```python
from build123d import *

# Parameters (mm, degrees)
SKETCH1_R             = 101
SKETCH1_R_2           = 3.175
SKETCH1_R_3           = 86.77
BOSS_EXTRUDE1_DEPTH   = 6
SKETCH1_R_4           = 84.23
SKETCH1_R_5           = 70
BOSS_EXTRUDE1_2_DEPTH = 6
SKETCH1_3_R           = 86.77
SKETCH1_3_R_2         = 84.23
BOSS_EXTRUDE2_DEPTH   = 1.5875
BOSS_EXTRUDE3_START   = 6
SKETCH1_4_R           = 84.23
SKETCH1_4_R_2         = 3.175
SKETCH1_4_R_3         = 70
BOSS_EXTRUDE3_DEPTH   = 2
BOSS_EXTRUDE4_START   = -8
SKETCH1_5_R           = 101
SKETCH1_5_R_2         = 3.175
SKETCH1_5_R_3         = 86.77
BOSS_EXTRUDE4_DEPTH   = 2


with BuildPart() as part:
    # Sketch1 → Boss-Extrude1 (new, symmetric)
    with BuildSketch(Plane(origin=(0, 0, 0), x_dir=(1, 0, 0), z_dir=(0, 1, 0))):
        with Locations(Location((0, 0, 0), (0, 0, 270))):
            Circle(SKETCH1_R)
        with Locations(Location((-66.888765966, -66.888765966, 0), (0, 0, 270))):
            Circle(SKETCH1_R_2, mode=Mode.SUBTRACT)
        with Locations(Location((66.888765966, 66.888765966, 0), (0, 0, 270))):
            Circle(SKETCH1_R_2, mode=Mode.SUBTRACT)
        with Locations(Location((0, 0, 0), (0, 0, 270))):
            Circle(SKETCH1_R_3, mode=Mode.SUBTRACT)
        with Locations(Location((66.888765966, -66.888765966, 0), (0, 0, 270))):
            Circle(SKETCH1_R_2, mode=Mode.SUBTRACT)
        with Locations(Location((-66.888765966, 66.888765966, 0), (0, 0, 270))):
            Circle(SKETCH1_R_2, mode=Mode.SUBTRACT)
    extrude(amount=BOSS_EXTRUDE1_DEPTH, both=True)



with BuildPart() as body_2:
    # Sketch1 → Boss-Extrude1 2 (new, symmetric)
    with BuildSketch(Plane(origin=(0, 0, 0), x_dir=(1, 0, 0), z_dir=(0, 1, 0))):
        with Locations(Location((0, 0, 0), (0, 0, 270))):
            Circle(SKETCH1_R_4)
        with Locations(Location((-54.800775542, 54.800775542, 0), (0, 0, 270))):
            Circle(SKETCH1_R_2, mode=Mode.SUBTRACT)
        with Locations(Location((-54.800775542, -54.800775542, 0), (0, 0, 270))):
            Circle(SKETCH1_R_2, mode=Mode.SUBTRACT)
        with Locations(Location((54.800775542, -54.800775542, 0), (0, 0, 270))):
            Circle(SKETCH1_R_2, mode=Mode.SUBTRACT)
        with Locations(Location((54.800775542, 54.800775542, 0), (0, 0, 270))):
            Circle(SKETCH1_R_2, mode=Mode.SUBTRACT)
        with Locations(Location((0, 0, 0), (0, 0, 270))):
            Circle(SKETCH1_R_5, mode=Mode.SUBTRACT)
    extrude(amount=BOSS_EXTRUDE1_2_DEPTH, both=True)


with BuildPart() as part_1:
    add(part.part)

    add(body_2.part)  # Boss-Extrude2 merges body 2
    # Sketch1<3> → Boss-Extrude2 (add, symmetric)
    with BuildSketch(Plane(origin=(0, 0, 0), x_dir=(1, 0, 0), z_dir=(0, 1, 0))):
        with Locations(Location((0, 0, 0), (0, 0, 270))):
            Circle(SKETCH1_3_R)
        with Locations(Location((0, 0, 0), (0, 0, 270))):
            Circle(SKETCH1_3_R_2, mode=Mode.SUBTRACT)
    extrude(amount=BOSS_EXTRUDE2_DEPTH, both=True)

    # Sketch1<4> → Boss-Extrude3 (add)
    with BuildSketch(Plane(origin=(0, 0, 0), x_dir=(1, 0, 0), z_dir=(0, 1, 0)).offset(BOSS_EXTRUDE3_START)):
        with Locations(Location((0, 0, 0), (0, 0, 270))):
            Circle(SKETCH1_4_R)
        with Locations(Location((-54.800775542, 54.800775542, 0), (0, 0, 270))):
            Circle(SKETCH1_4_R_2, mode=Mode.SUBTRACT)
        with Locations(Location((-54.800775542, -54.800775542, 0), (0, 0, 270))):
            Circle(SKETCH1_4_R_2, mode=Mode.SUBTRACT)
        with Locations(Location((54.800775542, -54.800775542, 0), (0, 0, 270))):
            Circle(SKETCH1_4_R_2, mode=Mode.SUBTRACT)
        with Locations(Location((54.800775542, 54.800775542, 0), (0, 0, 270))):
            Circle(SKETCH1_4_R_2, mode=Mode.SUBTRACT)
        with Locations(Location((0, 0, 0), (0, 0, 270))):
            Circle(SKETCH1_4_R_3, mode=Mode.SUBTRACT)
    extrude(amount=BOSS_EXTRUDE3_DEPTH)

    # Sketch1<5> → Boss-Extrude4 (add)
    with BuildSketch(Plane(origin=(0, 0, 0), x_dir=(1, 0, 0), z_dir=(0, 1, 0)).offset(BOSS_EXTRUDE4_START)):
        with Locations(Location((0, 0, 0), (0, 0, 270))):
            Circle(SKETCH1_5_R)
        with Locations(Location((-66.888765966, -66.888765966, 0), (0, 0, 270))):
            Circle(SKETCH1_5_R_2, mode=Mode.SUBTRACT)
        with Locations(Location((66.888765966, 66.888765966, 0), (0, 0, 270))):
            Circle(SKETCH1_5_R_2, mode=Mode.SUBTRACT)
        with Locations(Location((0, 0, 0), (0, 0, 270))):
            Circle(SKETCH1_5_R_3, mode=Mode.SUBTRACT)
        with Locations(Location((66.888765966, -66.888765966, 0), (0, 0, 270))):
            Circle(SKETCH1_5_R_2, mode=Mode.SUBTRACT)
        with Locations(Location((-66.888765966, 66.888765966, 0), (0, 0, 270))):
            Circle(SKETCH1_5_R_2, mode=Mode.SUBTRACT)
    extrude(amount=BOSS_EXTRUDE4_DEPTH)


solid = part_1.part
```
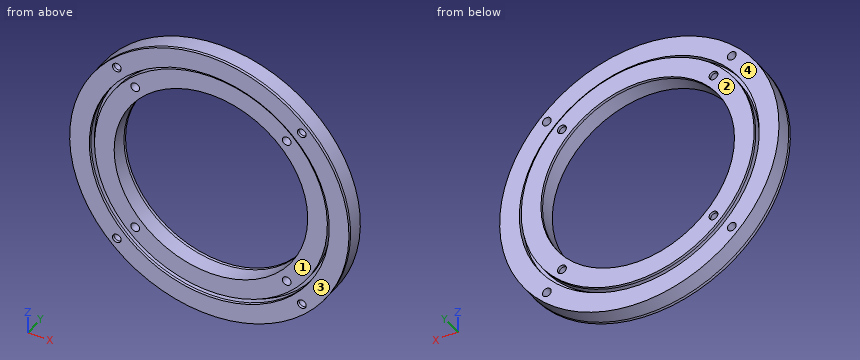
Model file for the job. Use its own axes, mm. Face numbers are marked on the shaded views. A direction names the side the tool comes from. Round coordinates to 2 decimals unless told otherwise and drop trailing zeros. Write each loop counter-clockwise with the first axis right and the second up, starting at its lowest first coordinate (ties: lowest second). Pieces come first, ordered by that corner, then holes. Notation, with made-up numbers: M -28.5,75 L 1.5,75 A13 cw 1.5,86 Z; hole C 2.25,-7 d3. An arc over 180 degrees is marked long. Put each result on its own line as item: value.
Item 1: Flat gauge pins, fed straight in: P1, Ø7.5, axis at x = 54.8, z = -54.8, coming from the +Y side; P2, Ø5, axis at x = -54.8, z = -54.8, coming from the -Y side; P3, Ø7.5, axis at x = 66.89, z = -66.89, coming from the +Y side; P4, Ø1, axis at x = 34.5, y = -3.5, coming from the +Z side. Where does each tip first touch, or does it go through?
Responses:
P1: y = 8
P2: through
P3: y = 6
P4: z = 95.11
Item 2: Mould opens along X. For the marked faces 1 and 2 say: +X half, -X half, draft (parallel to the pull), parting line (faces both ways), or undercut.
Responses:
face 1: undercut
face 2: draft
Item 3: Cut at B-B (x = 0). List the corners of the cut face in (y, z), and give its area (3 significant figures).
Responses:
outline: M -8,-101 L 6,-101 L 6,-86.77 L 1.59,-86.77 L 1.59,-84.23 L 8,-84.23 L 8,-70 L -6,-70 L -6,-84.23 L -1.59,-84.23 L -1.59,-86.77 L -8,-86.77 Z; M -8,86.77 L -1.59,86.77 L -1.59,84.23 L -6,84.23 L -6,70 L 8,70 L 8,84.23 L 1.59,84.23 L 1.59,86.77 L 6,86.77 L 6,101 L -8,101 Z
area: 813 mm²
Item 4: Cut at A-A (z = 0). List the corners of the cut face in (x, y).
Responses:
outline: M -101,-8 L -86.77,-8 L -86.77,-1.59 L -84.23,-1.59 L -84.23,-6 L -70,-6 L -70,8 L -84.23,8 L -84.23,1.59 L -86.77,1.59 L -86.77,6 L -101,6 Z; M 70,-6 L 84.23,-6 L 84.23,-1.59 L 86.77,-1.59 L 86.77,-8 L 101,-8 L 101,6 L 86.77,6 L 86.77,1.59 L 84.23,1.59 L 84.23,8 L 70,8 Z
Item 5: Tool access for the marked faces 3 and 4: list every direction of +Z, -Z, +X, -X, +Y, -Y with a clear straight run to the whole face (end or side of a thin tool).
Responses:
face 3: +Z, -Z, +X, -X, -Y
face 4: +Y
Item 6: Probe L1, parallel to X at y = 7.2, z = 0; L2, parallel to X at y = 6.5, z = -52; L3, parallel to Z at x = 16, y = 3.5. List the from-to ranges inside material, lowest first. Write a range as from..to.
Responses:
L1: -84.23..-70, 70..84.23
L2: -66.26..-56.3, -53.31..-46.86, 46.86..53.31, 56.3..66.26
L3: -99.72..-85.28, -82.7..-68.15, 68.15..82.7, 85.28..99.72
